from build123d import *

# Parameters (mm, degrees)
BOSS_EXTRU_1_DEPTH      = 57.5
ESQUISSE3_R             = 42.5
ENL_V_MAT_EXTRU_1_DEPTH = 50
ESQUISSE4_W             = 155
ESQUISSE4_H             = 116.672618896
BOSS_EXTRU_2_DEPTH      = 10
CHANFREIN1_SIZE         = 20
ENL_V_MAT_EXTRU_2_REACH = 163.73
ENL_V_START             = -10
ESQUISSE4_3_W           = 20
ESQUISSE4_3_H           = 96.672618896
CONG_3_R                = 5
CONG_1_R                = 4
CONG_2_R                = 5


with BuildPart() as part:
    # Esquisse2 → Boss.-Extru.1 (new, symmetric)
    with BuildSketch(Plane(origin=(0, 0, 0), x_dir=(0, 0, -1), z_dir=(1, 0, 0))):
        Polygon((8.838834765, 109.601551084), (15.909902577, 116.672618896), (58.336309448, 74.246212025), (58.336309448, 0), (-58.336309448, 0), (-58.336309448, 42.426406871), (-51.265241636, 49.497474683), (-15.909902577, 14.142135624), (44.194173824, 74.246212025), align=None)
        Polygon((-51.265241636, 49.497474683), (8.838834765, 109.601551084), (44.194173824, 74.246212025), (-15.909902577, 14.142135624), align=None)
    extrude(amount=BOSS_EXTRU_1_DEPTH, both=True)

    # Esquisse3 → Enlèv. mat.-Extru.1 (cut)
    with BuildSketch(Plane(origin=(0, 50.38135816, 50.38135816), x_dir=(1, 0, 0), z_dir=(0, 0.7071067811865441, 0.7071067811865509))):
        with Locations(Location((0, 41.25, 0), (0, 0, 270))):
            Circle(ESQUISSE3_R)
    extrude(amount=-ENL_V_MAT_EXTRU_1_DEPTH, mode=Mode.SUBTRACT)

    # Esquisse4 → Boss.-Extru.2 (add)
    with BuildSketch(Plane.XZ):
        Rectangle(ESQUISSE4_W, ESQUISSE4_H)
    extrude(amount=-BOSS_EXTRU_2_DEPTH)

    # Chanfrein1
    chanfrein1_edges = [part.edges().sort_by_distance(p)[0] for p in [
        (57.5, 10, 0),
        (-57.5, 10, 0),
    ]]
    chamfer(chanfrein1_edges, length=CHANFREIN1_SIZE - 0.0001)  # a hair under: the kernel refuses the full size

    # Esquisse4<3> → Enlèv. mat.-Extru.2 (cut, up to next)
    with BuildSketch(Plane.XZ.offset(ENL_V_START), mode=Mode.PRIVATE) as enl_v_mat_extru_2_sk1:
        with Locations((-67.5, 0)):
            Rectangle(ESQUISSE4_3_W, ESQUISSE4_3_H)
    enl_v_mat_extru_2_tool1 = extrude(enl_v_mat_extru_2_sk1.sketch, amount=-ENL_V_MAT_EXTRU_2_REACH, mode=Mode.PRIVATE) & part.part
    # Esquisse4<3> → Enlèv. mat.-Extru.2 (cut, up to next)
    with BuildSketch(Plane.XZ.offset(ENL_V_START), mode=Mode.PRIVATE) as enl_v_mat_extru_2_sk2:
        with Locations((67.5, 0)):
            Rectangle(ESQUISSE4_3_W, ESQUISSE4_3_H)
    enl_v_mat_extru_2_tool2 = extrude(enl_v_mat_extru_2_sk2.sketch, amount=-ENL_V_MAT_EXTRU_2_REACH, mode=Mode.PRIVATE) & part.part
    add(enl_v_mat_extru_2_tool1.solids().sort_by_distance((-67.5, 10, 0))[0], mode=Mode.SUBTRACT)
    add(enl_v_mat_extru_2_tool2.solids().sort_by_distance((67.5, 10, 0))[0], mode=Mode.SUBTRACT)

    # Congé3
    cong_3_edges = [part.edges().sort_by_distance(p)[0] for p in [
        (57.5, 29.9999, 53.336309448),
        (-57.5, 29.9999, -53.336309448),
        (-57.5, 29.9999, 53.336309448),
        (57.5, 29.9999, -53.336309448),
        (-57.5, 19.99995, 48.336309448),
        (-57.5, 10, 0),
        (-57.5, 19.99995, -48.336309448),
        (-67.49995, 10, 48.336309448),
        (-67.49995, 10, -48.336309448),
        (67.49995, 10, -48.336309448),
        (57.5, 19.99995, -48.336309448),
        (57.5, 10, 0),
        (67.49995, 10, 48.336309448),
        (57.5, 19.99995, 48.336309448),
    ]]
    fillet(cong_3_edges, radius=CONG_3_R)

    # Congé1
    cong_1_edges = [part.edges().sort_by_distance(p)[0] for p in [
        (0, 74.246212025, -44.194173824),
    ]]
    fillet(cong_1_edges, radius=CONG_1_R)

    # Congé2
    cong_2_edges = [part.edges().sort_by_distance(p)[0] for p in [
        (0, 74.246212025, -58.336309448),
        (57.5, 95.45941546, -37.123106012),
        (-77.5, 5, 58.336309448),
        (-77.5, 5, -58.336309448),
        (77.5, 5, 58.336309448),
        (77.5, 5, -58.336309448),
        (-57.5, 95.45941546, -37.123106012),
    ]]
    fillet(cong_2_edges, radius=CONG_2_R)


solid = part.part
Work out the finished part from the listing and answer in its coordinate system (mm). A direction names the side the tool comes from. Give positions to 0.01 mm unless a question says otherwise; leave off trailing zeros.
Q1. Given pin 1 (4.5 mm diameter, centred on x = 69.5, z = 0, fed in from +Y); pin 2 (16.5 mm diameter, centred on x = -68.5, z = -18.5, fed in from +Y); pin 3 (1 mm diameter, centred on y = 14.5, z = 18, fed in from +X); pin 4 (3 mm diameter, centred on x = -67, y = 21.5, fed in from +Z), each flat-ended and moving along its own axis, determine where each tip first touches the part or whether it passes through.
Answer:
pin 1: stops at y = 10
pin 2: stops at y = 10.53
pin 3: stops at x = 57.6
pin 4: stops at z = 58.34
Q2. For a pull along Z with two mould halves and no side action, classify faces 1 (the face through (0.73, 96.48, -36.1)), 2 (the face through (-68.1, 19.4, -52.6)), 3 (the face through (66, 19, 48.336)) as released by +Z, released by -Z, zero draft, split by the parting line, or undercut.
Answer:
face 1: released by -Z
face 2: zero draft
face 3: undercut
Q3. A tool of negligible diameter and unlimited length cuts with its end or side. For faces 4 (the face through (-68.1, 19.4, 52.4)), 5 (the face through (-57.5, 54, -1)), 6 (the face through (58.926, 21.758, 46.833)), from which of +Z, -Z, +X, -X, +Y, -Y can it reach the whole face along a straight path? Write none if from no direction.
Answer:
face 4: +Z, -Z, -X, +Y
face 5: -X, +Y
face 6: +X, +Y
Q4. Straight lines are drawn through the part: L1, parallel to X at y = 19, z = -31; L2, parallel to Y at x = -32, z = 39.5; L3, parallel to X at y = 84, z = -21. For each, find the intervals that lie inside material, in ascending order.
Answer:
L1: x = -57.5 to 57.5
L2: y = 0 to 58.28
L3: x = -57.5 to -26.79, 26.79 to 57.5
